Model file for the job. Use its own axes, mm. Coordinates: 2 decimals unless noted, no trailing zeros. Order: outer loops, then holes, each group sorted by start corner. A loop starts at its lowest first (then second) coordinate and runs counter-clockwise, first axis right, second up. Notation, with made-up numbers: (40, 31) - (90, 31) arc R28 cw to (90, 51) - close; hole circle Ø11 at (-6, -18.75). An arc over 180 degrees is marked (long way). Put each result on its own line as item: value. Start each with the question number.
Autodesk Inventor part; units mm, degrees
ref_plane "YZ Plane" through (0, 0, 0) normal (1, 0, 0) x (0, 1, 0)
ref_plane "XZ Plane" through (0, 0, 0) normal (0, 1, 0) x (-1, 0, 0)
ref_plane "XY Plane" through (0, 0, 0) normal (0, 0, 1) x (1, 0, 0)
sketch "Boceto1" plane through (0, 0, 0) normal (0, 1, 0) x (-1, 0, 0)
  line L0 (0, 0) -> (30, 0)
  line L1 (30, 0) -> (30, -375)
  line L2 (30, -375) -> (0, -375)
  line L3 (0, -375) -> (0, 0)
  circle A0 centre (15, -187.5) radius 4.5
  dimension "d0" = 375
  dimension "d1" = 30
  dimension "d4" = 9
  dimension "d5" = 15
  dimension "d6" = 187.5
extrude "Extrusión2" add sketch "Boceto1" along normal blind 5
properties part number "Base.pin.Seg" material "Acrílico, claro"
Item 1: Wall check: line 1 along Z through (x, y) = (-15.25, 1); line 2 along Z through (x, y) = (-18.5, 4.35). Give the ranges that are in metal, low to high.
Item 2: Pull direction Z, two halves, no side cores. Call faces 1 (the face through (-8, 0, -185)), 2 (the face through (-14.02, 2.46, -183.11)): pulls with the +Z half, pulls with the -Z half, needs draft (parallel to the pull), parting line crosses it, or undercut.
Item 3: Slice it at A-A, the plane x = -15. Give the cut face in (y, z), plus the area to 3 significant figures.
Item 4: Slice it at B-B, the plane z = -187.5. Give the cut face in (x, y), plus the area to 3 significant figures.
Item 5: Flat gauge pin, fed straight in: pin 1 Ø7 at (x, z) = (-15, -187.5) entering from +Y. Where does the tip first touch, or does it go through?
Here are the results:
1. line 1: z = -375 to -191.99, -183.01 to 0
1. line 2: z = -375 to -190.33, -184.67 to 0
2. face 1: needs draft
2. face 2: undercut
3. outline: (0, -375) - (5, -375) - (5, -192) - (0, -192) - close; (0, -183) - (5, -183) - (5, 0) - (0, 0) - close
3. area: 1,830 mm^2
4. outline: (-30, 0) - (-19.5, 0) - (-19.5, 5) - (-30, 5) - close; (-10.5, 0) - (0, 0) - (0, 5) - (-10.5, 5) - close
4. area: 105 mm^2
5. pin 1: passes through
